```python
from build123d import *

# Parameters (mm, degrees)
BOSS_EXTRUDE1_DEPTH = 2
SKETCH2_W           = 122.7
SKETCH2_H           = 1.5
BOSS_EXTRUDE2_DEPTH = 3
CUT_EXTRUDE1_DEPTH  = 0.25
BOSS_EXTRUDE3_START = 4.25
BOSS_EXTRUDE3_DEPTH = 4.25
SKETCH5_R           = 1.175
CUT_EXTRUDE2_DEPTH  = 68.954676991


with BuildPart() as part:
    # Sketch1 → Boss-Extrude1 (new body)
    with BuildSketch(Plane(origin=(0, 0, 0), x_dir=(1, 0, 0), z_dir=(0, 1, 0))):
        Polygon((-61.35, 26.875), (-48.84, 26.875), (-48.84, 28.875), (-38.84, 28.875), (-38.84, 26.875), (-3.84, 26.875), (-3.84, 28.875), (6.16, 28.875), (6.16, 26.875), (41.16, 26.875), (41.16, 28.875), (51.16, 28.875), (51.16, 26.875), (61.35, 26.875), (61.35, -26.875), (51.16, -26.875), (51.16, -28.875), (41.16, -28.875), (41.16, -26.875), (6.16, -26.875), (6.16, -28.875), (-3.84, -28.875), (-3.84, -26.875), (-38.84, -26.875), (-38.84, -28.875), (-48.84, -28.875), (-48.84, -26.875), (-61.35, -26.875), align=None)
    extrude(amount=BOSS_EXTRUDE1_DEPTH)

    # Sketch2 → Boss-Extrude2 (add)
    with BuildSketch(Plane(origin=(0, 2, 0), x_dir=(1, 0, 0), z_dir=(0, 1, 0))):
        with Locations((0, 26.125)):
            Rectangle(SKETCH2_W, SKETCH2_H)
        with Locations((0, -26.125)):
            Rectangle(SKETCH2_W, SKETCH2_H)
    extrude(amount=BOSS_EXTRUDE2_DEPTH)

    # Sketch3 → Cut-Extrude1 (cut)
    with BuildSketch(Plane(origin=(0, 2, 0), x_dir=(1, 0, 0), z_dir=(0, 1, 0))):
        with BuildLine():
            Line((-35.55, 22.15), (55.85, 22.15))
            ThreePointArc((55.85, 22.15), (56.910660172, 21.710660172), (57.35, 20.65))
            Line((57.35, 20.65), (57.35, -20.65))
            ThreePointArc((57.35, -20.65), (56.910660172, -21.710660172), (55.85, -22.15))
            Line((55.85, -22.15), (-35.55, -22.15))
            ThreePointArc((-35.55, -22.15), (-36.610660172, -21.710660172), (-37.05, -20.65))
            Line((-37.05, -20.65), (-37.05, 20.65))
            ThreePointArc((-37.05, 20.65), (-36.610660172, 21.710660172), (-35.55, 22.15))
        make_face()
    extrude(amount=-CUT_EXTRUDE1_DEPTH, mode=Mode.SUBTRACT)

    # Sketch4 → Boss-Extrude3 (add)
    with BuildSketch(Plane(origin=(0, 2, 0), x_dir=(1, 0, 0), z_dir=(0, 1, 0)).offset(BOSS_EXTRUDE3_START)):
        with BuildLine():
            Line((55.85, 23.4), (-35.55, 23.4))
            ThreePointArc((-35.55, 23.4), (-37.494543648, 22.594543648), (-38.3, 20.65))
            Line((-38.3, 20.65), (-38.3, -20.65))
            ThreePointArc((-38.3, -20.65), (-37.494543648, -22.594543648), (-35.55, -23.4))
            Line((-35.55, -23.4), (55.85, -23.4))
            ThreePointArc((55.85, -23.4), (57.794543648, -22.594543648), (58.6, -20.65))
            Line((58.6, -20.65), (58.6, 20.65))
            ThreePointArc((58.6, 20.65), (57.794543648, 22.594543648), (55.85, 23.4))
        make_face()
        with BuildLine():
            Line((55.85, 22.15), (-35.55, 22.15))
            ThreePointArc((-35.55, 22.15), (-36.610660172, 21.710660172), (-37.05, 20.65))
            Line((-37.05, 20.65), (-37.05, -20.65))
            ThreePointArc((-37.05, -20.65), (-36.610660172, -21.710660172), (-35.55, -22.15))
            Line((-35.55, -22.15), (55.85, -22.15))
            ThreePointArc((55.85, -22.15), (56.910660172, -21.710660172), (57.35, -20.65))
            Line((57.35, -20.65), (57.35, 20.65))
            ThreePointArc((57.35, 20.65), (56.910660172, 21.710660172), (55.85, 22.15))
        make_face(mode=Mode.SUBTRACT)
    extrude(amount=-BOSS_EXTRUDE3_DEPTH)

    # Sketch5 → Cut-Extrude2 (cut, through all)
    with BuildSketch(Plane(origin=(0, 1.75, 0), x_dir=(1, 0, 0), z_dir=(0, 1, 0))):
        with Locations(Location((-32.35, 17.2, 0), (0, 0, 270))):
            Circle(SKETCH5_R)
        with Locations(Location((52.65, 17.2, 0), (0, 0, 270))):
            Circle(SKETCH5_R)
        with Locations(Location((52.65, -17.2, 0), (0, 0, 270))):
            Circle(SKETCH5_R)
        with Locations(Location((-32.35, -17.2, 0), (0, 0, 270))):
            Circle(SKETCH5_R)
    extrude(amount=-CUT_EXTRUDE2_DEPTH, mode=Mode.SUBTRACT)


solid = part.part
```
Can you work these out from the model? Positions are in its coordinate system, mm. A direction names the side the tool comes from. Round coordinates to 2 decimals unless told otherwise and drop trailing zeros. Loops run counter-clockwise (first coordinate to the right, second up) from the corner with the lowest first, then second, coordinate; pieces in that order, holes last. Notation, with made-up numbers: M -11.5,7.5 L 0.5,7.5 A8 ccw 0.5,13.5 Z; hole C 2,78.5 d10. An arc over 180 degrees is marked long. Answer in a Markdown table with one row per item.
1. If we section it at C-C, the plane x = 52.65: Please give me the cut outline in (y, z) (3 decimals).
Established:
| item | result |
|---|---|
| outline | M 0,-26.875 L 5,-26.875 L 5,-25.375 L 2,-25.375 L 2,-23.4 L 6.25,-23.4 L 6.25,-22.15 L 1.75,-22.15 L 1.75,-18.375 L 0,-18.375 Z; M 0,-16.025 L 1.75,-16.025 L 1.75,16.025 L 0,16.025 Z; M 0,18.375 L 1.75,18.375 L 1.75,22.15 L 6.25,22.15 L 6.25,23.4 L 2,23.4 L 2,25.375 L 5,25.375 L 5,26.875 L 0,26.875 Z |
2. Please list where these lines run through material, in increasing order: line 1 (X direction, y = 1.1, z = 17.2) (3 decimals); line 2 (Z direction, x = -2, y = 4) (3 decimals); line 3 (X direction, y = 2.25, z = -16.5). Write a range as from..to.
Established:
| item | result |
|---|---|
| line 1 | -61.35..-33.525, -31.175..51.475, 53.825..61.35 |
| line 2 | -26.875..-25.375, -23.4..-22.15, 22.15..23.4, 25.375..26.875 |
| line 3 | -38.3..-37.05, 57.35..58.6 |
3. On a 3-axis mill with a long thin cutter (end or side, diameter ignored), from which of +Z, -Z, +X, -X, +Y, -Y can I reach the whole of each face in a straight line? I mean faces 4 (the face through (10, 4, 22.15)), 5 (the face through (57.77, 4.15, 22.62)), 6 (the face through (-37.47, 4.15, -22.62)). Say none if no direction works.
Established:
| item | result |
|---|---|
| face 4 | +Y |
| face 5 | +X, +Y |
| face 6 | -X, +Y |
4. If we section it at B-B, the plane z = 17.2: Please give me the cut outline in (x, y) (3 decimals).
Established:
| item | result |
|---|---|
| outline | M -61.35,0 L -33.525,0 L -33.525,1.75 L -37.05,1.75 L -37.05,6.25 L -38.3,6.25 L -38.3,2 L -61.35,2 Z; M -31.175,0 L 51.475,0 L 51.475,1.75 L -31.175,1.75 Z; M 53.825,0 L 61.35,0 L 61.35,2 L 58.6,2 L 58.6,6.25 L 57.35,6.25 L 57.35,1.75 L 53.825,1.75 Z |
5. Thinking about a two-plate mould opening in Z: for faces 1 (the face through (11, 1.75, 0)), 2 (the face through (61.35, 1, 0)), 3 (the face through (-38.3, 4, 0)), which applies, pulls with the +Z half, pulls with the -Z half, needs draft (parallel to the pull), parting line crosses it, or undercut?
Established:
| item | result |
|---|---|
| face 1 | undercut |
| face 2 | needs draft |
| face 3 | undercut |
6. If we section it at A-A, the plane y = 3: Please give me the cut outline in (x, z) (3 decimals).
Established:
| item | result |
|---|---|
| outline | M -61.35,-26.875 L 61.35,-26.875 L 61.35,-25.375 L -61.35,-25.375 Z; M -61.35,25.375 L 61.35,25.375 L 61.35,26.875 L -61.35,26.875 Z; M -38.3,-20.65 A2.75 ccw -35.55,-23.4 L 55.85,-23.4 A2.75 ccw 58.6,-20.65 L 58.6,20.65 A2.75 ccw 55.85,23.4 L -35.55,23.4 A2.75 ccw -38.3,20.65 Z; hole M -37.05,-20.65 A1.5 ccw -35.55,-22.15 L 55.85,-22.15 A1.5 ccw 57.35,-20.65 L 57.35,20.65 A1.5 ccw 55.85,22.15 L -35.55,22.15 A1.5 ccw -37.05,20.65 Z |
7. I'm going to push flat-ended pins straight in: pin 1 Ø8 at (x, z) = (46, -3.5) entering from +Y; pin 2 Ø0.6 at (x, z) = (1, -27.5) entering from +Y; pin 3 Ø1.3 at (y, z) = (5, -7.5) entering from +X; pin 4 Ø1.9 at (x, z) = (-32.35, -17.2) entering from -Y. Where does each tip first touch, or does it pass through?
Established:
| item | result |
|---|---|
| pin 1 | y = 1.75 |
| pin 2 | y = 2 |
| pin 3 | x = 58.6 |
| pin 4 | through |
8. If we section it at D-D, the plane x = 25: Please give me the cut outline in (y, z) (3 decimals), plus the area to 3 significant figures.
Established:
| item | result |
|---|---|
| outline | M 0,-26.875 L 5,-26.875 L 5,-25.375 L 2,-25.375 L 2,-23.4 L 6.25,-23.4 L 6.25,-22.15 L 1.75,-22.15 L 1.75,22.15 L 6.25,22.15 L 6.25,23.4 L 2,23.4 L 2,25.375 L 5,25.375 L 5,26.875 L 0,26.875 Z |
| area | 116 mm² |
